The listing builds one solid part. Answer for the finished solid, in the listing's coordinates (mm). A direction names the side the tool comes from. Coordinates: 2 decimals unless noted, no trailing zeros. Order: outer loops, then holes, each group sorted by start corner. A loop starts at its lowest first (then second) coordinate and runs counter-clockwise, first axis right, second up.
from build123d import *

# Parameters (mm, degrees)
SKETCH_1_W      = 14.849242405
SKETCH_1_H      = 14.849242405
EXTRUDE_6_DEPTH = 15
SKETCH_4_W      = 13
SKETCH_4_H      = 13
EXTRUDE_7_DEPTH = 80


with BuildPart() as part:
    # 草图1 → 凸台-拉伸6 (new body)
    with BuildSketch(Plane.XY):
        with Locations((-32.575378798, 32.575378798)):
            Rectangle(SKETCH_1_W, SKETCH_1_H)
        Polygon((25.150757595, 40), (-25.150757595, 40), (-25.150757595, 25.150757595), (-40, 25.150757595), (-40, -25.150757595), (-25.150757595, -25.150757595), (-25.150757595, -40), (25.150757595, -40), (25.150757595, -25.150757595), (40, -25.150757595), (40, 25.150757595), (25.150757595, 25.150757595), align=None)
        with Locations((32.575378798, 32.575378798)):
            Rectangle(SKETCH_1_W, SKETCH_1_H)
        Polygon((40, -39.62158524), (40, -25.150757595), (25.150757595, -25.150757595), (25.150757595, -40), (39.62158524, -40), (40, -40), align=None)
        Polygon((-25.150757595, -25.150757595), (-40, -25.150757595), (-40, -40), (-25.902864758, -40), (-25.150757595, -40), align=None)
    extrude(amount=EXTRUDE_6_DEPTH)

    # 草图4 → 凸台-拉伸7 (add)
    with BuildSketch(Plane.XY.offset(15)):
        with Locations((-33.5, 33.5)):
            Rectangle(SKETCH_4_W, SKETCH_4_H)
        with Locations((33.5, 33.5)):
            Rectangle(SKETCH_4_W, SKETCH_4_H)
        with Locations((-33.5, -33.5)):
            Rectangle(SKETCH_4_W, SKETCH_4_H)
        with Locations((33.5, -33.5)):
            Rectangle(SKETCH_4_W, SKETCH_4_H)
    extrude(amount=EXTRUDE_7_DEPTH)


solid = part.part
(1) Find section A-A on z = 40.5. Determine the outline of the cut face in (x, y), then the cut area to 3 significant figures.
(2) Find the intervals of material crossed by probe 1 along X at (y, z) = (-30, 32); probe 2 along Z at (x, y) = (-7, -15), in increasing order.
(3) Given pin 1 Ø1 at (x, y) = (27.5, -16) entering from +Z, flat-ended and moving along its own axis, determine where the tip first touches the part or whether it passes through.
(4) Find section C-C on x = -22.5. Determine the outline of the cut face in (y, z), then the cut area to 3 significant figures.
(5) The mould has two halves that part along Y. Classify faces 4 (the flat face through (-1, 1, 15)), 5 (the flat face through (27, 33, 54)), 6 (the flat face through (-27.2, 40, 36.3)): pulls with the +Y half, pulls with the -Y half, needs draft (parallel to the pull), parting line crosses it, or undercut.
(6) A tool of negligible diameter and unlimited length cuts with its end or side. For faces 1 (the flat face through (-34, -27, 54)), 2 (the flat face through (-27, -34, 54)), 3 (the flat face through (-34, -33, 95)), from which of +Z, -Z, +X, -X, +Y, -Y can it reach the whole face along a straight path? Write none if from no direction.
(7) Find section B-B on y = 30. Determine the outline of the cut face in (x, z), then the cut area to 3 significant figures.
Resolved:
1. outline: (-40, -40) - (-27, -40) - (-27, -27) - (-40, -27) - close; (-40, 27) - (-27, 27) - (-27, 40) - (-40, 40) - close; (27, -40) - (40, -40) - (40, -27) - (27, -27) - close; (27, 27) - (40, 27) - (40, 40) - (27, 40) - close
1. area: 676 mm2
2. probe 1: x = -40 to -27, 27 to 40
2. probe 2: z = 0 to 15
3. pin 1: stops at z = 15
4. outline: (-40, 0) - (40, 0) - (40, 15) - (-40, 15) - close
4. area: 1,200 mm2
5. face 4: undercut
5. face 5: needs draft
5. face 6: pulls with the +Y half
6. face 1: +Z, +X, -X
6. face 2: +Z, +Y, -Y
6. face 3: +Z, +X, -X, +Y, -Y
7. outline: (-40, 0) - (40, 0) - (40, 95) - (27, 95) - (27, 15) - (-27, 15) - (-27, 95) - (-40, 95) - close
7. area: 3,280 mm2
